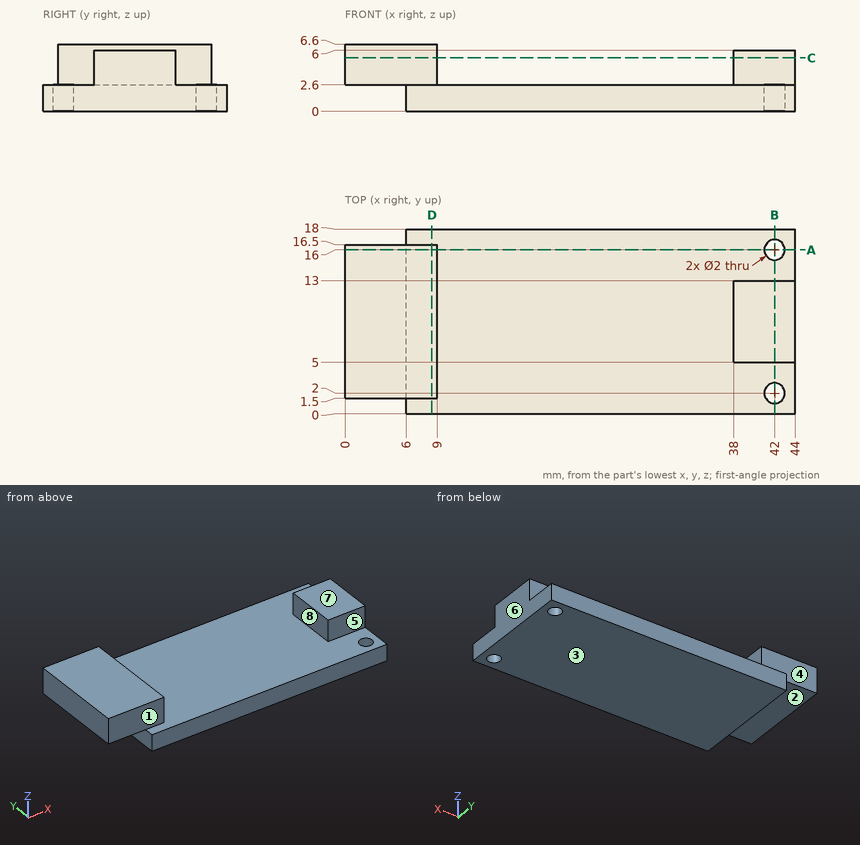
Input: dimensioned drawing with shaded views. Units: mm. Origin: part minimum x, y, z. A direction names the side the tool comes from. Coordinates: 2 decimals unless noted, no trailing zeros. Order: outer loops, then holes, each group sorted by start corner. A loop starts at its lowest first (then second) coordinate and runs counter-clockwise, first axis right, second up.
Item 1: Section query C-C (z = 5.25). Output: boundary loops of the cut face in (x, y), then the cut area to 3 significant figures.
Answer:
outline: (0, 1.5) - (9, 1.5) - (9, 16.5) - (0, 16.5) - close; (38, 5) - (44, 5) - (44, 13) - (38, 13) - close
area: 183 mm2
Item 2: Draft query along X for the marked faces 6, 7 and 8. Return one class per face: released by +X, released by -X, zero draft, split by the parting line, or undercut.
Answer:
face 6: released by +X
face 7: zero draft
face 8: undercut
Item 3: Material intervals for line 1 along Y through (x, z) = (42, 1.9); line 2 along X through (y, z) = (12.5, 4); line 3 along Z through (x, y) = (20, 14.25), sorted ascending.
Answer:
line 1: y = 0 to 1, 3 to 15, 17 to 18
line 2: x = 0 to 9, 38 to 44
line 3: z = 0 to 2.6
Item 4: Contact query for flat-ended pins moving along their axis: P1, Ø1.7, axis at x = 40.5, z = 4.5, coming from the +Y side; P2, Ø5, axis at x = 19.5, y = 12, coming from the +Z side; P3, Ø1.8, axis at x = 40.5, y = 9, coming from the +Z side; P4, Ø1.8, axis at x = 42, y = 2, coming from the -Z side. Output: stop coordinate, or through.
Answer:
P1: stops at y = 13
P2: stops at z = 2.6
P3: stops at z = 6
P4: passes through
Item 5: Section query A-A (y = 16). Output: boundary loops of the cut face in (x, z), then the cut area to 3 significant figures.
Answer:
outline: (0, 2.6) - (6, 2.6) - (6, 0) - (41, 0) - (41, 2.6) - (9, 2.6) - (9, 6.6) - (0, 6.6) - close; (43, 0) - (44, 0) - (44, 2.6) - (43, 2.6) - close
area: 130 mm2
Item 6: Section query D-D (x = 8.5). Output: boundary loops of the cut face in (y, z), then the cut area to 3 significant figures.
Answer:
outline: (0, 0) - (18, 0) - (18, 2.6) - (16.5, 2.6) - (16.5, 6.6) - (1.5, 6.6) - (1.5, 2.6) - (0, 2.6) - close
area: 107 mm2
Item 7: Access query for the marked faces 1, 2, 3, 4 and 5. Directions: +Z, -Z, +X, -X, +Y, -Y. A direction counts if a zero-diameter tool reaches every point of the face in a straight line with its end or side. Return the directions, or none.
Answer:
face 1: +Z, +X, -X, -Y
face 2: -Z, -X, +Y, -Y
face 3: -Z, +X, -X, +Y, -Y
face 4: +Z, +X, -X, +Y
face 5: +Z, +X, -Y
Item 8: Section query B-B (x = 42). Output: boundary loops of the cut face in (y, z).
Answer:
outline: (0, 0) - (1, 0) - (1, 2.6) - (0, 2.6) - close; (3, 0) - (15, 0) - (15, 2.6) - (13, 2.6) - (13, 6) - (5, 6) - (5, 2.6) - (3, 2.6) - close; (17, 0) - (18, 0) - (18, 2.6) - (17, 2.6) - close
